Here's how the part is built. I have some questions about the finished solid (model axes, mm). A direction names the side the tool comes from. Give positions to 0.01 mm unless a question says otherwise; leave off trailing zeros. Loops run counter-clockwise (first coordinate to the right, second up) from the corner with the lowest first, then second, coordinate; pieces in that order, holes last.
Q1. I need wall thicknesses on line 1 (X direction, y = 8.5, z = -3.25); line 2 (Y direction, x = -171.5, z = -5.5) (1 decimal); line 3 (X direction, y = 9, z = -3.5). Which ranges of each line are inside material? Lowest first, please.
Q2. If we section it at A-A (y = 0): Please give me the cut outline in (x, z).
Q3. We'd pull the mould along Y, two halves only. Please class faces 1 (the face through (169, 60.325, -3)), 2 (the face through (185.817, 47.265, -3.131)): +Y half, -Y half, draft (parallel to the pull), parting line (faces both ways), or undercut.
Q4. Will these pins go through, and if not, where does the flat tip stop? P1, Ø2.5, axis at y = -21.5, z = -4, coming from the -X side; P2, Ø2, axis at y = -13.5, z = -4, coming from the +X side; P3, Ø1, axis at y = -5, z = -3, coming from the -X side.
Q5. If we section it at D-D (x = -53): Please give me the cut outline in (y, z), plus the area to 3 significant figures.
Q6. For faces 3 (the face through (-185.82, -25.04, -3.13)), 4 (the face through (190.5, -30, -5)), 5 (the face through (-194, 55.562, -3)), which set-ups out of +Z, -Z, +X, -X, +Y, -Y let a thin tool reach every point of the face, with its end or its side?
Q7. If we section it at C-C (y = 42): Please give me the cut outline in (x, z).
from build123d import *

# Parameters (mm, degrees)
SKETCH1_W                      = 6.35
SKETCH1_H                      = 4.7625
SKETCH1_R                      = 12.7
SKETCH1_R_2                    = 6.35
BOSS_EXTRUDE1_DEPTH            = 6.35
SKETCH2_W                      = 6.35
SKETCH2_H                      = 9.525
BOSS_EXTRUDE2_DEPTH            = 6.35
FILLET1_R                      = 12.7
FILLET2_R                      = 11.1125
F_6_32_TAPPED_HOLE1_D          = 2.7051
F_6_32_TAPPED_HOLE1_DEPTH      = 9.398
F_6_32_TAPPED_HOLE1_TIP        = 0.81269403
FILLET3_R                      = 9.525
FILLET4_R                      = 12.7
F_6_32_TAPPED_HOLE2_AT_2_COUNT = 2
F_6_32_TAPPED_HOLE2_AT_2_PITCH = 79.375
FILLET5_R                      = 3.175


with BuildPart() as part:
    # Sketch1 → Boss-Extrude1 (new body)
    # profile 1 of 11: a face of its own
    with BuildSketch(Plane.XY):
        with Locations((-193.675, -35.71875)):
            Rectangle(SKETCH1_W, SKETCH1_H)
    # profile 2 of 11: a face of its own
    with BuildSketch(Plane.XY):
        with Locations((-193.675, 57.94375)):
            Rectangle(SKETCH1_W, SKETCH1_H)
    # profile 3 of 11: a face of its own
    with BuildSketch(Plane.XY):
        with BuildLine():
            Line((-190.5, 55.5625), (-139.7, 55.5625))
            ThreePointArc((-139.7, 55.5625), (-127.904529217, 55.251640636), (-116.141805402, 54.31992556))
            ThreePointArc((-116.141805402, 54.31992556), (-58.142540048, 40.183298939), (-5.938839164, 11.225871431))
            ThreePointArc((-5.938839164, 11.225871431), (-3.059528789, 12.325959743), (0, 12.7))
            ThreePointArc((0, 12.7), (-65.90259045, 48.091568013), (-139.7, 60.325))
            Line((-139.7, 60.325), (-190.5, 60.325))
            Line((-190.5, 60.325), (-190.5, 55.5625))
        make_face()
    # profile 4 of 11: a face of its own
    with BuildSketch(Plane.XY):
        with BuildLine():
            ThreePointArc((-139.7, 55.5625), (-95.25, 11.1125), (-139.7, -33.3375))
            Line((-139.7, -33.3375), (-118.579686171, -33.3375))
            ThreePointArc((-118.579686171, -33.3375), (-90.506521339, 9.744357657), (-116.141805402, 54.31992556))
            ThreePointArc((-116.141805402, 54.31992556), (-127.904529217, 55.251640636), (-139.7, 55.5625))
        make_face()
    # profile 5 of 11: a face of its own
    with BuildSketch(Plane.XY):
        Polygon((190.5, -38.1), (190.5, -33.3375), (-118.579686171, -33.3375), (-190.5, -33.3375), (-190.5, -38.1), align=None)
    # profile 6 of 11: a face of its own
    with BuildSketch(Plane.XY):
        Circle(SKETCH1_R)
        Circle(SKETCH1_R_2, mode=Mode.SUBTRACT)
    # profile 7 of 11: a face of its own
    with BuildSketch(Plane.XY):
        with BuildLine():
            Line((-2.38125, -33.3375), (2.38125, -33.3375))
            Line((2.38125, -33.3375), (2.38125, -12.474760456))
            ThreePointArc((2.38125, -12.474760456), (0, -12.7), (-2.38125, -12.474760456))
            Line((-2.38125, -12.474760456), (-2.38125, -33.3375))
        make_face()
    # profile 8 of 11: a face of its own
    with BuildSketch(Plane.XY):
        with BuildLine():
            ThreePointArc((116.141805402, 54.31992556), (127.904529217, 55.251640636), (139.7, 55.5625))
            Line((139.7, 55.5625), (190.5, 55.5625))
            Line((190.5, 55.5625), (190.5, 60.325))
            Line((190.5, 60.325), (139.7, 60.325))
            ThreePointArc((139.7, 60.325), (65.90259045, 48.091568013), (0, 12.7))
            ThreePointArc((0, 12.7), (3.059528789, 12.325959743), (5.938839164, 11.225871431))
            ThreePointArc((5.938839164, 11.225871431), (58.142540048, 40.183298939), (116.141805402, 54.31992556))
        make_face()
    # profile 9 of 11: a face of its own
    with BuildSketch(Plane.XY):
        with BuildLine():
            Line((118.579686171, -33.3375), (139.7, -33.3375))
            ThreePointArc((139.7, -33.3375), (95.25, 11.1125), (139.7, 55.5625))
            ThreePointArc((139.7, 55.5625), (127.904529217, 55.251640636), (116.141805402, 54.31992556))
            ThreePointArc((116.141805402, 54.31992556), (90.506521339, 9.744357657), (118.579686171, -33.3375))
        make_face()
    # profile 10 of 11: a face of its own
    with BuildSketch(Plane.XY):
        with Locations((193.675, 57.94375)):
            Rectangle(SKETCH1_W, SKETCH1_H)
    # profile 11 of 11: a face of its own
    with BuildSketch(Plane.XY):
        with Locations((193.675, -35.71875)):
            Rectangle(SKETCH1_W, SKETCH1_H)
    extrude(amount=-BOSS_EXTRUDE1_DEPTH)

    # Sketch2 → Boss-Extrude2 (add)
    with BuildSketch(Plane.XY):
        with Locations((-187.325, -28.575)):
            Rectangle(SKETCH2_W, SKETCH2_H)
        with Locations((-187.325, 50.8)):
            Rectangle(SKETCH2_W, SKETCH2_H)
        with Locations((187.325, 50.8)):
            Rectangle(SKETCH2_W, SKETCH2_H)
        with Locations((187.325, -28.575)):
            Rectangle(SKETCH2_W, SKETCH2_H)
    extrude(amount=-BOSS_EXTRUDE2_DEPTH)

    # Fillet1
    # the kernel refuses this fillet: 12.7 mm, written as the material it adds along each edge
    with BuildSketch(Plane(origin=(184.15, -33.3375, 0), x_dir=(-1, 0, 0), z_dir=(0, 0, -1)), Plane(origin=(-184.15, 55.5625, 0), x_dir=(1, 0, 0), z_dir=(0, 0, -1))) as fillet1_piece_1:
        with BuildLine():
            CenterArc((12.296722124, 12.7), FILLET1_R, 194.477512186, 75.522487814)
            Line((0, 9.525), (-0.245934442, 9.4615))
            ThreePointArc((-0.245934442, 9.4615), (-0.254, 4.7625), (-0.254, 0))
            Line((-0.254, 0), (0, -0.254))
            Line((0, -0.254), (12.296722124, -0.254))
            Line((12.296722124, -0.254), (12.296722124, 0))
        make_face()
    extrude(amount=6.35)
    with BuildSketch(Plane(origin=(184.15, 55.5625, 0), x_dir=(-1, 0, 0), z_dir=(0, 0, -1)), Plane(origin=(-184.15, -33.3375, 0), x_dir=(1, 0, 0), z_dir=(0, 0, -1))) as fillet1_piece_2:
        with BuildLine():
            CenterArc((12.296722124, -12.7), FILLET1_R, 90, 75.522487814)
            Line((0, -9.525), (-0.245934442, -9.4615))
            ThreePointArc((-0.245934442, -9.4615), (-0.254, -4.7625), (-0.254, 0))
            Line((-0.254, 0), (0, 0.254))
            Line((0, 0.254), (12.296722124, 0.254))
            Line((12.296722124, 0.254), (12.296722124, 0))
        make_face()
    extrude(amount=6.35)

    # Fillet2
    # the kernel refuses this fillet: 11.1125 mm, written as the material it takes off along each edge
    with BuildSketch(Plane(origin=(184.15, -23.8125, 15.875), x_dir=(1, 0, 0), z_dir=(0, 0, -1))) as fillet2_piece_1:
        with BuildLine():
            CenterArc((6.758920293, 11.10497368), FILLET2_R, 216.847264444, 51.043876357)
            Line((-2.133712835, 4.440985963), (-2.311565498, 4.307706209))
            ThreePointArc((-2.311565498, 4.307706209), (-1.049758647, 2.228707764), (-0.215192637, -0.0555625))
            Line((-0.215192637, -0.0555625), (0, -0.22225))
            ThreePointArc((0, -0.22225), (3.175, -0.22225), (6.341821594, -0.222099474))
            Line((6.341821594, -0.222099474), (6.35, 0))
        make_face()
    extrude(amount=38.1, mode=Mode.SUBTRACT)
    with BuildSketch(Plane(origin=(184.15, 46.0375, 15.875), x_dir=(-0.43306748122172517, 0.9013615016785834, 0), z_dir=(0, 0, -1))) as fillet2_piece_2:
        with BuildLine():
            CenterArc((7.082527166, 10.901433526), FILLET2_R, 207.771247513, 51.043876357)
            Line((-2.749978506, 5.723645536), (-2.946628619, 5.620089776))
            ThreePointArc((-2.946628619, 5.620089776), (-1.575316847, 2.76557352), (-0.200327594, -0.096249248))
            Line((-0.200327594, -0.096249248), (0.043111035, -0.218028671))
            ThreePointArc((0.043111035, -0.218028671), (2.46348771, 0.018968828), (4.883864385, -0.218028671))
            Line((4.883864385, -0.218028671), (4.92697542, 0))
        make_face()
    extrude(amount=38.1, mode=Mode.SUBTRACT)
    with BuildSketch(Plane(origin=(-184.15, -23.8125, 15.875), x_dir=(-1, 0, 0), z_dir=(0, 0, -1))) as fillet2_piece_3:
        with BuildLine():
            CenterArc((6.758920293, -11.10497368), FILLET2_R, 92.108859198, 51.043876357)
            Line((-2.133712835, -4.440985963), (-2.311565498, -4.307706209))
            ThreePointArc((-2.311565498, -4.307706209), (-1.049758647, -2.228707764), (-0.215192637, 0.0555625))
            Line((-0.215192637, 0.0555625), (0, 0.22225))
            ThreePointArc((0, 0.22225), (3.175, 0.22225), (6.341821594, 0.222099474))
            Line((6.341821594, 0.222099474), (6.35, 0))
        make_face()
    extrude(amount=38.1, mode=Mode.SUBTRACT)
    with BuildSketch(Plane(origin=(-184.15, 46.0375, 15.875), x_dir=(0.43306748122172517, 0.9013615016785834, 0), z_dir=(0, 0, -1))) as fillet2_piece_4:
        with BuildLine():
            CenterArc((7.082527166, -10.901433526), FILLET2_R, 101.184876129, 51.043876357)
            Line((-2.749978506, -5.723645536), (-2.946628619, -5.620089776))
            ThreePointArc((-2.946628619, -5.620089776), (-1.575316847, -2.76557352), (-0.200327594, 0.096249248))
            Line((-0.200327594, 0.096249248), (0.043111035, 0.218028671))
            ThreePointArc((0.043111035, 0.218028671), (2.46348771, -0.018968828), (4.883864385, 0.218028671))
            Line((4.883864385, 0.218028671), (4.92697542, 0))
        make_face()
    extrude(amount=38.1, mode=Mode.SUBTRACT)

    # #6-32 Tapped Hole1
    with Locations(Plane(origin=(0, -38.1, 0), x_dir=(-1, 0, 0), z_dir=(0, -1, 0))):
        with Locations((82.55, 3.175)):
            Hole(F_6_32_TAPPED_HOLE1_D / 2, depth=F_6_32_TAPPED_HOLE1_DEPTH)
            with Locations((0, 0, -(F_6_32_TAPPED_HOLE1_DEPTH + F_6_32_TAPPED_HOLE1_TIP / 2))):  # 118° drill point
                Cone(0, F_6_32_TAPPED_HOLE1_D / 2, F_6_32_TAPPED_HOLE1_TIP, mode=Mode.SUBTRACT)

    # Fillet3
    fillet3_edges = [part.edges().sort_by_distance(p)[0] for p in [
        (2.38125, -12.474760456, -3.175),
        (2.38125, -33.3375, -3.175),
        (5.938839164, 11.225871431, -3.175),
        (-2.38125, -33.3375, -3.175),
        (-2.38125, -12.474760456, -3.175),
        (-5.938839164, 11.225871431, -3.175),
    ]]
    fillet(fillet3_edges, radius=FILLET3_R)

    # Fillet4
    fillet4_edges = [part.edges().sort_by_distance(p)[0] for p in [
        (0, 12.7, -3.175),
    ]]
    fillet(fillet4_edges, radius=FILLET4_R)

    # Sketch12 → #6-32 Tapped Hole2 (revolve, cut)
    with BuildSketch(Plane(origin=(190.5, -28.575, -3.175), x_dir=(0, 0, -1), z_dir=(0, 1, 0))):
        Polygon((0, 0), (0, 10.21069403), (1.35255, 9.398), (1.35255, 7.112), (1.7526, 7.112), (1.7526, 0), align=None)
    f_6_32_tapped_hole2 = revolve(axis=Axis((196.85, -28.575, -3.175), (-1, 0, 0)), mode=Mode.SUBTRACT)

    # #6-32 Tapped Hole2 at 2: #6-32 Tapped Hole2 ×2
    with Locations(*[(0, i * F_6_32_TAPPED_HOLE2_AT_2_PITCH, 0) for i in range(1, F_6_32_TAPPED_HOLE2_AT_2_COUNT)]):
        add(f_6_32_tapped_hole2, mode=Mode.SUBTRACT)

    # Mirror1: #6-32 Tapped Hole2 across plane
    add(f_6_32_tapped_hole2.mirror(Plane(origin=(0, 0, 0), x_dir=(0, 0, 1), z_dir=(1, 0, 0))), mode=Mode.SUBTRACT)

    # Mirror1 copy 1 sketch → Mirror1 copy 1 (revolve, cut)
    with BuildSketch(Plane(origin=(-190.5, 50.8, -3.175), x_dir=(0, 0, -1), z_dir=(0, 1, 0))):
        Polygon((0, 0), (0, -10.21069403), (1.35255, -9.398), (1.35255, -7.112), (1.7526, -7.112), (1.7526, 0), align=None)
    revolve(axis=Axis((-196.85, 50.8, -3.175), (-1, 0, 0)), mode=Mode.SUBTRACT)

    # Fillet5
    fillet5_edges = [part.edges().sort_by_distance(p)[0] for p in [
        (118.579686171, -33.3375, -3.175),
        (116.141805402, 54.31992556, -3.175),
        (-116.141805402, 54.31992556, -3.175),
        (-118.579686171, -33.3375, -3.175),
    ]]
    fillet(fillet5_edges, radius=FILLET5_R)


solid = part.part
Check sheet entries:
1. line 1: x = -95.33 to -90.56, -10.6 to 10.6, 90.56 to 95.33
1. line 2: y = -38.1 to -33.3, 55.6 to 60.3
1. line 3: x = -95.3 to -90.53, -10.56 to 10.56, 90.53 to 95.3
2. outline: (-96.66, -6.35) - (-91.76, -6.35) - (-91.76, 0) - (-96.66, 0) - close; (-12.7, -6.35) - (-6.35, -6.35) - (-6.35, 0) - (-12.7, 0) - close; (6.35, -6.35) - (12.7, -6.35) - (12.7, 0) - (6.35, 0) - close; (91.76, -6.35) - (96.66, -6.35) - (96.66, 0) - (91.76, 0) - close
3. face 1: +Y half
3. face 2: undercut
4. P1: stops at x = -110.91
4. P2: stops at x = 103.37
4. P3: stops at x = -98.47
5. outline: (-38.1, -6.35) - (-33.34, -6.35) - (-33.34, 0) - (-38.1, 0) - close; (38.1, -6.35) - (43.25, -6.35) - (43.25, 0) - (38.1, 0) - close
5. area: 63.0 mm2
6. face 3: +Z, -Z
6. face 4: +Z, -Z, +X
6. face 5: +Z, -Z, -X
7. outline: (-107.73, -6.35) - (-101.39, -6.35) - (-101.39, 0) - (-107.73, 0) - close; (-62.95, -6.35) - (-50, -6.35) - (-50, 0) - (-62.95, 0) - close; (50, -6.35) - (62.95, -6.35) - (62.95, 0) - (50, 0) - close; (101.39, -6.35) - (107.73, -6.35) - (107.73, 0) - (101.39, 0) - close
